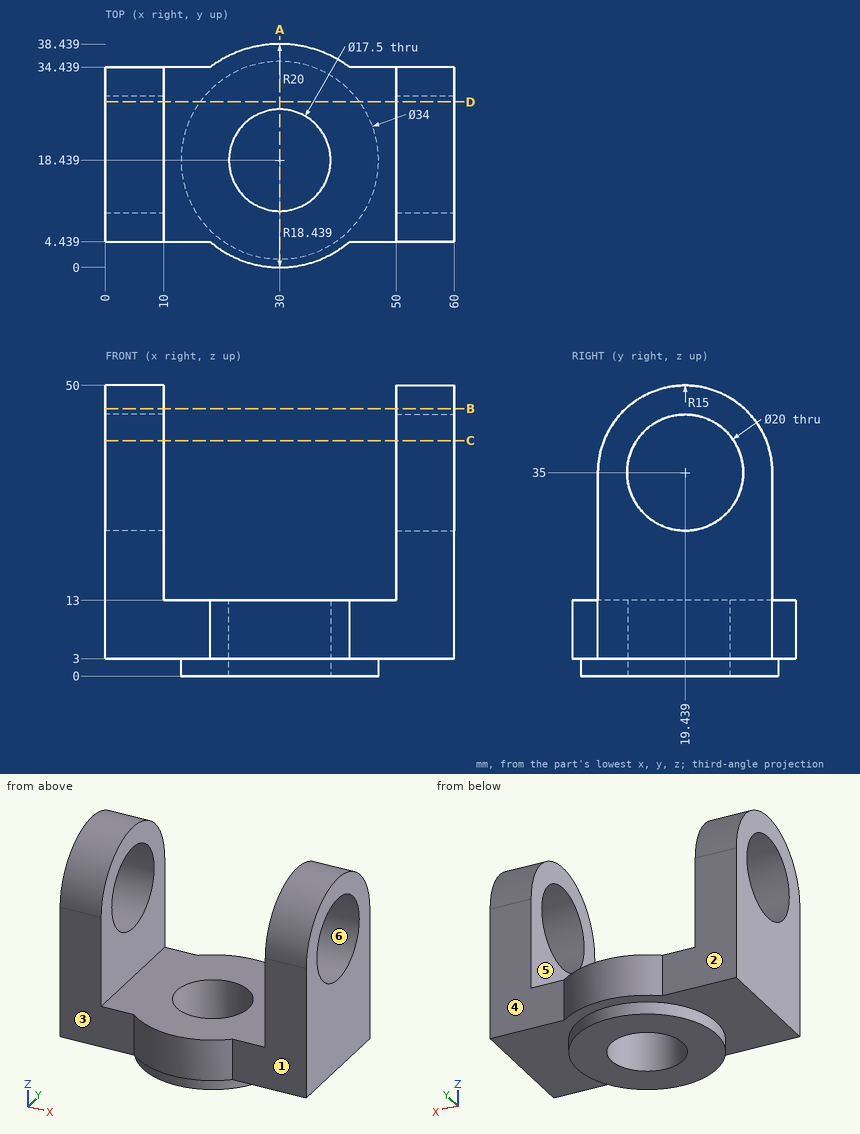
The drawing under review shows one solid part. Ordinate dimensions are in mm from its lowest x, y, z. A direction names the side the tool comes from. Coordinates: 2 decimals unless noted, no trailing zeros. Order: outer loops, then holes, each group sorted by start corner. A loop starts at its lowest first (then second) coordinate and runs counter-clockwise, first axis right, second up. Notation, with made-up numbers: (-7.5, 49.25) -> (1.5, 49.25) arc R32 cw to (1.5, 79.25) -> close; hole circle Ø9 at (89, 61.25). An arc over 180 degrees is marked (long way). Return JSON: item names as keys, results as strings.
1. The part is to be moulded in two halves that separate along Y. For the marked faces 4, 5 and 6, say which applies: +Y half, -Y half, draft (parallel to the pull), parting line (faces both ways), or undercut.
Answer block:
{"face 4": "+Y half", "face 5": "draft", "face 6": "undercut"}
2. We need section A-A on x = 30. Write out the cut boundary in (y, z), and give its area (3 significant figures).
Answer block:
{"outline": "(0, 3) -> (1.44, 3) -> (1.44, 0) -> (9.69, 0) -> (9.69, 13) -> (0, 13) -> close; (27.19, 0) -> (35.44, 0) -> (35.44, 3) -> (38.44, 3) -> (38.44, 13) -> (27.19, 13) -> close", "area": "259 mm²"}
3. For pin 1 Ø14.5 at (x, z) = (9.5, 15) entering from +Y; pin 2 Ø6 at (x, y) = (20.5, 14.5) entering from +Z; pin 3 Ø20 at (x, z) = (11, 24.5) entering from -Y, all flat-tipped, find the tip position at first contact; note any pin that passes through.
Answer block:
{"pin 1": "y = 34.44", "pin 2": "z = 13", "pin 3": "y = 4.44"}
4. We need section B-B on z = 46. Write out the cut boundary in (x, y), and give its area (3 significant figures).
Answer block:
{"outline": "(0, 9.24) -> (10, 9.24) -> (10, 29.64) -> (0, 29.64) -> close; (50, 9.24) -> (60, 9.24) -> (60, 29.64) -> (50, 29.64) -> close", "area": "408 mm²"}
5. We need section C-C on z = 40.5. Write out the cut boundary in (x, y).
Answer block:
{"outline": "(0, 5.48) -> (10, 5.48) -> (10, 11.09) -> (0, 11.09) -> close; (0, 27.79) -> (10, 27.79) -> (10, 33.39) -> (0, 33.39) -> close; (50, 5.48) -> (60, 5.48) -> (60, 11.09) -> (50, 11.09) -> close; (50, 27.79) -> (60, 27.79) -> (60, 33.39) -> (50, 33.39) -> close"}
6. Machinability: for the marked faces 1, 2 and 3, which of the approach directions +Z, -Z, +X, -X, +Y, -Y give a long, thin tool a straight path to every point of the face, cutting with its end or side? Answer none if there is none.
Answer block:
{"face 1": "+Z, -Z, +X, -Y", "face 2": "+Z, -Z, -X, +Y", "face 3": "+Z, -Z, -X, -Y"}
7. We need section D-D on y = 28.5. Write out the cut boundary in (x, z).
Answer block:
{"outline": "(0, 3) -> (16.3, 3) -> (16.3, 0) -> (43.7, 0) -> (43.7, 3) -> (60, 3) -> (60, 30.77) -> (50, 30.77) -> (50, 13) -> (10, 13) -> (10, 30.77) -> (0, 30.77) -> close; (0, 39.23) -> (10, 39.23) -> (10, 46.95) -> (0, 46.95) -> close; (50, 39.23) -> (60, 39.23) -> (60, 46.95) -> (50, 46.95) -> close"}
8. For line 1 (X direction, y = 29, z = 30); line 2 (Z direction, x = 44.5, y = 7.5); line 3 (Y direction, x = 54.5, z = 8), list the stretches that pass through material, from the lowest coordinate up. Write a range as from..to.
Answer block:
{"line 1": "0..10, 50..60", "line 2": "3..13", "line 3": "4.44..34.44"}
